from build123d import *

# Parameters (mm, degrees)
F0_W     = 540
F0_H     = 390
F1_DEPTH = 10
F2_W     = 80
F2_H     = 80
F2_R     = 15
F3_DEPTH = 10
F4_R     = 15
F5_DEPTH = 10
F6_DEPTH = 10
F7_DEPTH = 10


with BuildPart() as f1:
    # F0 (on Front) → F1 (new body)
    with BuildSketch(Plane.XZ):
        Polygon((-575.5810141563, 243.9473703504), (-465.5810141563, -206.0526296496), (133.660423523, -206.0526296496), (243.660423523, 243.9473703504), (133.660423523, 243.9473703504), (-465.5810141563, 243.9473703504), align=None)
        with Locations((-166.339576477, 18.9473703504)):
            Rectangle(F0_W, F0_H, mode=Mode.SUBTRACT)
        Polygon((-495.5810141563, 43.0153865893), (-537.3643879646, 213.9473703504), (-495.5810141563, 213.9473703504), align=None, mode=Mode.SUBTRACT)
        Polygon((163.660423523, 213.9473703504), (205.4437973313, 213.9473703504), (163.660423523, 43.0153865893), align=None, mode=Mode.SUBTRACT)
    extrude(amount=F1_DEPTH)

    # F2 (on face) → F3 (join)
    with BuildSketch(Plane.XZ.offset(10)):
        with Locations((-396.339576477, 173.9473703504)):
            Rectangle(F2_W, F2_H)
        with Locations((-396.339576477, 198.8157841563)):
            Circle(F2_R, mode=Mode.SUBTRACT)
        with Locations((63.660423523, 173.9473703504)):
            Rectangle(F2_W, F2_H)
        with Locations((63.660423523, 198.8157841563)):
            Circle(F2_R, mode=Mode.SUBTRACT)
        with Locations((63.660423523, -136.0526296496)):
            Rectangle(F2_W, F2_H)
        with Locations((63.660423523, -136.0526296496)):
            Circle(F2_R, mode=Mode.SUBTRACT)
        with Locations((-396.339576477, -136.0526296496)):
            Rectangle(F2_W, F2_H)
        with Locations((-396.339576477, -136.0526296496)):
            Circle(F2_R, mode=Mode.SUBTRACT)
    extrude(amount=-F3_DEPTH)

    # F4 (on face) → F5 (join)
    with BuildSketch(Plane.XZ.offset(10)):
        Polygon((243.660423523, 243.9473703504), (-575.5810141563, 243.9473703504), (-465.5810141563, -206.0526296496), (133.660423523, -206.0526296496), align=None)
        with Locations((-396.339576477, -136.0526296496)):
            Circle(F4_R, mode=Mode.SUBTRACT)
        Polygon((23.660423523, -96.0526296496), (23.660423523, -176.0526296496), (-356.339576477, -176.0526296496), (-356.339576477, -96.0526296496), (-436.339576477, -96.0526296496), (-436.339576477, 133.9473703504), (-356.339576477, 133.9473703504), (-356.339576477, 213.9473703504), (23.660423523, 213.9473703504), (23.660423523, 133.9473703504), (103.660423523, 133.9473703504), (103.660423523, -96.0526296496), align=None, mode=Mode.SUBTRACT)
        with Locations((63.660423523, -136.0526296496)):
            Circle(F4_R, mode=Mode.SUBTRACT)
        Polygon((-495.5810141563, 213.9473703504), (-495.5810141563, 43.0153865893), (-537.3643879646, 213.9473703504), align=None, mode=Mode.SUBTRACT)
        with Locations((-396.339576477, 198.8157841563)):
            Circle(F4_R, mode=Mode.SUBTRACT)
        Polygon((163.660423523, 43.0153865893), (163.660423523, 213.9473703504), (205.4437973313, 213.9473703504), align=None, mode=Mode.SUBTRACT)
        with Locations((63.660423523, 198.8157841563)):
            Circle(F4_R, mode=Mode.SUBTRACT)
        Polygon((-356.339576477, -176.0526296496), (23.660423523, -176.0526296496), (23.660423523, -96.0526296496), (103.660423523, -96.0526296496), (103.660423523, 133.9473703504), (23.660423523, 133.9473703504), (23.660423523, 213.9473703504), (-356.339576477, 213.9473703504), (-356.339576477, 133.9473703504), (-436.339576477, 133.9473703504), (-436.339576477, -96.0526296496), (-356.339576477, -96.0526296496), align=None)
        Polygon((-537.3643879646, 213.9473703504), (-495.5810141563, 43.0153865893), (-495.5810141563, 213.9473703504), align=None)
        Polygon((205.4437973313, 213.9473703504), (163.660423523, 213.9473703504), (163.660423523, 43.0153865893), align=None)
        with Locations((63.660423523, 198.8157841563)):
            Circle(F4_R)
        with Locations((-396.339576477, 198.8157841563)):
            Circle(F4_R)
        with Locations((-396.339576477, -136.0526296496)):
            Circle(F4_R)
        with Locations((63.660423523, -136.0526296496)):
            Circle(F4_R)
    extrude(amount=-F5_DEPTH)

    # F6 (add): a face of the model
    f6_faces = [f1.faces().sort_by_distance(p)[0] for p in [
        (-520.5810141563, -5, 18.9473703504),
    ]]
    extrude(f6_faces, amount=F6_DEPTH)

    # F7 (add): a face of the model
    f7_faces = [f1.faces().sort_by_distance(p)[0] for p in [
        (188.660423523, -5, 18.9473703504),
    ]]
    extrude(f7_faces, amount=F7_DEPTH)


solid = f1.part
The listing builds one solid part. Answer for the finished solid, in the listing's coordinates (mm). Coordinates: 2 decimals unless noted, no trailing zeros. Order: outer loops, then holes, each group sorted by start corner. A loop starts at its lowest first (then second) coordinate and runs counter-clockwise, first axis right, second up. Notation, with made-up numbers: (69, 1) -> (125, 1) arc R14 cw to (125, 8) -> close; hole circle Ø4 at (18.5, 24). An arc over 180 degrees is marked (long way). Answer in a Markdown table with one row per item. Add a question column.
Item 1: Find section B-B (z = -21.5). Write down the section's boundary in (x, y).
Item 2: Find the intervals of material crossed by L1, parallel to Z at x = -276, y = -3; L2, parallel to X at y = -4.75, z = 7.5; L3, parallel to X at y = -4.75, z = 125, in increasing order. Write a range as from..to.
Item 3: Find section A-A (y = -5.5). Write down the section's boundary in (x, z) (3 decimals), then the cut area to 3 significant figures.
Item 4: Find section C-C (x = 170.5). Write down the section's boundary in (y, z), then the cut area to 3 significant figures.
Item 5: Each of these flat-tipped pins is pushed along its axis until it touches: P1, Ø4, axis at y = -6.5, z = -121.5, coming from the -X side; P2, Ø2, axis at y = -5.5, z = 121, coming from the -X side; P3, Ø5, axis at x = -85.5, y = -7.5, coming from the -Z side. Where does it stop, or does it pass through?
Result set:
| question | item | result |
|---|---|---|
| 1 | outline | (-520.99, -10) -> (189.07, -10) -> (189.07, 0) -> (-520.99, 0) -> close |
| 2 | L1 | z = -206.05..243.95 |
| 2 | L2 | x = -528.08..196.16 |
| 2 | L3 | x = -556.8..224.88 |
| 3 | outline | (-585.295, 241.573) -> (-475.295, -208.427) -> (-465.581, -206.053) -> (133.66, -206.053) -> (143.374, -208.427) -> (253.374, 241.573) -> (243.66, 243.947) -> (-575.581, 243.947) -> close |
| 3 | area | 328,000 mm² |
| 4 | outline | (-10, -97.46) -> (0, -97.46) -> (0, 243.95) -> (-10, 243.95) -> close |
| 4 | area | 3,410 mm² |
| 5 | P1 | stops at x = -497.03 |
| 5 | P2 | stops at x = -556.07 |
| 5 | P3 | stops at z = -206.05 |
